Autodesk Fusion 360 part; units mm, degrees
sketch "Sketch1" plane through (0, 0, 0) normal (0, 1, 0) x (1, 0, 0)
  line L0 (0, 0) -> (18.3, 0)
  line L1 (18.3, 0) -> (18.3, -5)
  line L2 (18.3, -5) -> (0, -5)
  line L3 (0, -5) -> (0, 0)
  dimension "d1" = 18.3
  dimension "d2" = 5
extrude "Extrude1" add sketch "Sketch1" along normal blind 3
sketch "Sketch2" plane through (0, 3, 0) normal (0, 1, 0) x (-1, 0, 0)
  line L0 (0, 5) -> (-18.3, 5)
  line L1 (-18.3, 5) -> (-18.3, 0)
  line L2 (-18.3, 0) -> (0, 0)
  line L3 (0, 0) -> (0, 5)
  line L4 (0, 0) -> (-3, 0)
  line L5 (-3, 0) -> (-3, 5)
  line L6 (-3, 5) -> (0, 5)
  line L7 (0, 5) -> (0, 0)
  line L8 (-18.3, 0) -> (-15.3, 0)
  line L9 (-15.3, 0) -> (-15.3, 5)
  line L10 (-15.3, 5) -> (-18.3, 5)
  line L11 (-18.3, 5) -> (-18.3, 0)
  dimension "d5" = 3
  dimension "d6" = 3
  dimension "d7" = 5
extrude "Extrude2" add sketch "Sketch2" along normal blind 9 contours L0 L2 L3 L4 L5 L6 L7 | L0 L1 L2 L8 L9 L10 L11
fillet "Fillet1" radius 2 1 edges at (15.3, 3, 2.5)
fillet "Fillet2" radius 1 4 edges at (0, 0, 2.5) (18.3, 0, 2.5) (0, 12, 2.5) (18.3, 12, 2.5)
extrude "Extrude3" add 1 faces at (6.4333, 0, 1.6667) along direction (0, -1, 0) blind 4
sketch "Sketch3" plane through (17.3, 0, 0) normal (1, 0, 0) x (0, 0, -1)
  line L0 (0, 0) -> (-5, 0)
  line L1 (-5, 0) -> (-5, -4)
  line L2 (-5, -4) -> (0, -4)
  line L3 (0, -4) -> (0, 0)
  line L4 (-2.5, 0) -> (-2.5, -4) construction
  spline S0 degree 5 poles (-5, 0) (-4.9471, -0.0246) (-4.844, -0.0733) (-4.6979, -0.1449) (-4.5202, -0.2376) (-4.3258, -0.349) (-4.157, -0.4565) (-4.0094, -0.5614) (-3.8742, -0.666) (-3.7405, -0.7738) (-3.6051, -0.8883) (-3.4674, -1.0128) (-3.3291, -1.1499) (-3.192, -1.3006) (-3.0571, -1.4644) (-2.9245, -1.6395) (-2.7947, -1.8235) (-2.6678, -2.0138) (-2.5446, -2.208) (-2.4267, -2.4046) (-2.316, -2.6025) (-2.2148, -2.8012) (-2.1251, -3.0004) (-2.0487, -3.1999) (-1.9864, -3.3996) (-1.9389, -3.5995) (-1.9129, -3.7596) (-1.9, -3.8798) (-1.8945, -3.9599) (-1.8924, -4) knots 0 0 0 0 0 0 0.04 0.08 0.12 0.16 0.2 0.24 0.28 0.32 0.36 0.4 0.44 0.48 0.52 0.56 0.6 0.64 0.68 0.72 0.76 0.8 0.84 0.88 0.92 0.96 1 1 1 1 1 1
  line L5 (-4.3837, -0.2829) -> (-3.5871, -0.8801)
  point P0 (-3.9854, -0.5815)
  point P1 (-3.3558, -1.126)
  point P2 (-2.6836, -1.992)
  point P3 (-2.1229, -3.0139)
extrude "Extrude4" cut sketch "Sketch3" against normal blind 68 contours L1 L2 S0
extrude "Extrude5" add 1 faces at (6.4333, -4, 0.6308) along direction (0, -1, 0) blind 2
fillet "Fillet3" radius 0.5 1 edges at (9.15, -6, 1.8924)
equation "d1 = 12.3 mm + 6 mm"
Here's how the part is built. I have some questions about the finished solid (model axes, mm). A direction names the side the tool comes from. Round coordinates to 2 decimals unless told otherwise and drop trailing zeros. Order: outer loops, then holes, each group sorted by start corner. A loop starts at its lowest first (then second) coordinate and runs counter-clockwise, first axis right, second up. Notation, with made-up numbers: (55.5, 7) -> (99.5, 7) arc R9 ccw to (99.5, 20) -> close; hole circle Ø7 at (-23, 81). An arc over 180 degrees is marked (long way). Use a Markdown table: item, result. Add a question column.
(1) Suppose I cut it at D-D, the plane y = 4.5. Please give me the cut outline in (x, z).
(2) If we mould it in two halves opening along X, with no side actions, what happens to faces 4 (the face through (3, 7, 2)), 5 (the face through (17.999, 11.715, 2.465)), 6 (the face through (0, 6, 3))? For each: released by +X, released by -X, zero draft, split by the parting line, or undercut.
(3) Suppose I cut it at A-A, the plane y = 9.5. Please give me the cut outline in (x, z).
(4) For faces 1 (the face through (14.7, 3.57, 2.54)), 2 (the face through (9, -5, 1.892)), 3 (the face through (9, -6, 1)), which set-ups out of +Z, -Z, +X, -X, +Y, -Y let a thin tool reach every point of the face, with its end or its side?
(5) I need wall thicknesses on line 1 along X through (y, z) = (10.25, 4.6); line 2 along Y through (x, z) = (8, 0.5); line 3 along Y through (x, z) = (8.25, 2.1). Which ranges of each line are inside material? Lowest first, please.
(6) Suppose I cut it at B-B, the plane z = 1.1. Please give me the cut outline in (x, y), and give its area (3 significant figures).
(7) Suppose I cut it at C-C, the plane y = -4.25. Please give me the cut outline in (x, z), and give its area (3 significant figures).
(8) For pin 1 Ø3 at (y, z) = (-2, 3.5) entering from +X; pin 2 Ø0.9 at (y, z) = (-5, 1) entering from -X; pin 3 Ø2 at (x, z) = (9.5, 4) entering from +Y, each with a flat end and sliding along its axis, tell me the tip position at first contact or that it passes through.
Verdict:
| question | item | result |
|---|---|---|
| 1 | outline | (0, 0) -> (3, 0) -> (3, 5) -> (0, 5) -> close; (15.24, 0) -> (18.3, 0) -> (18.3, 5) -> (15.24, 5) -> close |
| 2 | face 4 | undercut |
| 2 | face 5 | released by +X |
| 2 | face 6 | released by -X |
| 3 | outline | (0, 0) -> (3, 0) -> (3, 5) -> (0, 5) -> close; (15.3, 0) -> (18.3, 0) -> (18.3, 5) -> (15.3, 5) -> close |
| 4 | face 1 | +Z, -Z, +Y |
| 4 | face 2 | +Z, +X, -X, -Y |
| 4 | face 3 | +Z, -Z, +X, -X, -Y |
| 5 | line 1 | 0 to 3, 15.3 to 18.3 |
| 5 | line 2 | -6 to 3 |
| 5 | line 3 | -3.07 to 3 |
| 6 | outline | (0, 1) arc R1 ccw to (1, 0) -> (1, -6) -> (17.3, -6) -> (17.3, 0) arc R1 ccw to (18.3, 1) -> (18.3, 11) arc R1 ccw to (17.3, 12) -> (15.3, 12) -> (15.3, 5) arc R2 cw to (13.3, 3) -> (3, 3) -> (3, 12) -> (1, 12) arc R1 ccw to (0, 11) -> close |
| 6 | area | 207 mm2 |
| 7 | outline | (1, 0) -> (17.3, 0) -> (17.3, 1.89) -> (1, 1.89) -> close |
| 7 | area | 30.8 mm2 |
| 8 | pin 1 | x = 17.3 |
| 8 | pin 2 | x = 1 |
| 8 | pin 3 | y = 3 |
